from build123d import *

# Parameters (mm, degrees)
MODEL_R             = 2.5
BOSS_EXTRUDE1_DEPTH = 3


with BuildPart() as part:
    # Model → Boss-Extrude1 (new body)
    with BuildSketch(Plane.XY):
        with BuildLine():
            Line((-36.75, 0), (36.75, 0))
            ThreePointArc((36.75, 0), (40.285533906, 1.464466094), (41.75, 5))
            Line((41.75, 5), (41.75, 15))
            ThreePointArc((41.75, 15), (40.285533906, 18.535533906), (36.75, 20))
            Line((36.75, 20), (16.321067812, 20))
            ThreePointArc((16.321067812, 20), (14.40765065, 20.380602337), (12.785533906, 21.464466094))
            Line((12.785533906, 21.464466094), (3.214466094, 31.035533906))
            ThreePointArc((3.214466094, 31.035533906), (2.130602337, 32.65765065), (1.75, 34.571067812))
            Line((1.75, 34.571067812), (1.75, 45.428932188))
            ThreePointArc((1.75, 45.428932188), (2.130602337, 47.34234935), (3.214466094, 48.964466094))
            Line((3.214466094, 48.964466094), (12.785533906, 58.535533906))
            ThreePointArc((12.785533906, 58.535533906), (14.40765065, 59.619397663), (16.321067812, 60))
            Line((16.321067812, 60), (36.75, 60))
            ThreePointArc((36.75, 60), (40.285533906, 61.464466094), (41.75, 65))
            Line((41.75, 65), (41.75, 75))
            ThreePointArc((41.75, 75), (40.285533906, 78.535533906), (36.75, 80))
            Line((36.75, 80), (2.371320344, 80))
            ThreePointArc((2.371320344, 80), (1.797295195, 80.114180701), (1.310660172, 80.439339828))
            Line((1.310660172, 80.439339828), (-17.810660172, 99.560660172))
            ThreePointArc((-17.810660172, 99.560660172), (-18.135819299, 100.047295195), (-18.25, 100.621320344))
            Line((-18.25, 100.621320344), (-18.25, 123.5))
            ThreePointArc((-18.25, 123.5), (-18.689339828, 124.560660172), (-19.75, 125))
            Line((-19.75, 125), (-36.75, 125))
            ThreePointArc((-36.75, 125), (-37.810660172, 124.560660172), (-38.25, 123.5))
            Line((-38.25, 123.5), (-38.25, 1.5))
            ThreePointArc((-38.25, 1.5), (-37.810660172, 0.439339828), (-36.75, 0))
        make_face()
        with Locations((-28.25, 70)):
            Circle(MODEL_R, mode=Mode.SUBTRACT)
        with Locations((-8.25, 30)):
            Circle(MODEL_R, mode=Mode.SUBTRACT)
        with Locations((-8.25, 50)):
            Circle(MODEL_R, mode=Mode.SUBTRACT)
        with Locations((11.75, 70)):
            Circle(MODEL_R, mode=Mode.SUBTRACT)
        with Locations((31.75, 70)):
            Circle(MODEL_R, mode=Mode.SUBTRACT)
        with Locations((31.75, 10)):
            Circle(MODEL_R, mode=Mode.SUBTRACT)
        with Locations((11.75, 10)):
            Circle(MODEL_R, mode=Mode.SUBTRACT)
        with Locations((-28.25, 10)):
            Circle(MODEL_R, mode=Mode.SUBTRACT)
        with Locations((-28.25, 110)):
            Circle(MODEL_R, mode=Mode.SUBTRACT)
        with BuildLine():
            Line((-34.25, 119.15), (-34.25, 117.03))
            ThreePointArc((-34.25, 117.03), (-33.828233765, 116.011766235), (-32.81, 115.59))
            Line((-32.81, 115.59), (-23.69, 115.59))
            ThreePointArc((-23.69, 115.59), (-22.671766235, 116.011766235), (-22.25, 117.03))
            Line((-22.25, 117.03), (-22.25, 119.15))
            ThreePointArc((-22.25, 119.15), (-22.671766235, 120.168233765), (-23.69, 120.59))
            Line((-23.69, 120.59), (-32.81, 120.59))
            ThreePointArc((-32.81, 120.59), (-33.828233765, 120.168233765), (-34.25, 119.15))
        make_face(mode=Mode.SUBTRACT)
    extrude(amount=BOSS_EXTRUDE1_DEPTH)


solid = part.part
Geometry: final body of the model. Coordinates: model frame, mm. A direction names the side the tool comes from. Round coordinates to 2 decimals unless told otherwise and drop trailing zeros. Order: outer loops, then holes, each group sorted by start corner. A loop starts at its lowest first (then second) coordinate and runs counter-clockwise, first axis right, second up. Notation, with made-up numbers: (-34, -28.75) - (-13, -28.75) arc R11 ccw to (-13, -16.75) - close; hole circle Ø11 at (-36, 43.5). An arc over 180 degrees is marked (long way). Write each question's results on one line, items separated by ' | '.
Item 1: First-contact query: pin 1 Ø4 at (x, y) = (-28.25, 10) entering from -Z; pin 2 Ø1.5 at (x, z) = (17, 2) entering from +Y. Flat tips, straight axial feed; report the tip coordinate or a pass-through.
Completed:
pin 1: through | pin 2: y = 80
Item 2: Mould query, pull axis Y, two halves, no side actions, for faces 1 (the flat face through (-38.25, 63, 1)), 2 (the flat face through (-28, 125, 1)), 3 (the cylindrical face through (-8.79, 47.56, 1.48)). Classes: pulls with the +Y half, pulls with the -Y half, needs draft (parallel to the pull), parting line crosses it, or undercut.
Completed:
face 1: needs draft | face 2: pulls with the +Y half | face 3: undercut
Item 3: Material intervals for line 1 along Y through (x, z) = (31.75, 1.6); line 2 along X through (y, z) = (118.5, 0.3); line 3 along Y through (x, z) = (-24.5, 1.45), sorted ascending. Write a range as [from, to].
Completed:
line 1: [0, 7.5], [12.5, 20], [60, 67.5], [72.5, 80] | line 2: [-38.25, -34.25], [-22.25, -18.25] | line 3: [0, 115.59], [120.59, 125]
Item 4: Section A-A, the plane x = 26.5. Return the cut outline in (y, z), and give its area (3 significant figures).
Completed:
outline: (0, 0) - (20, 0) - (20, 3) - (0, 3) - close; (60, 0) - (80, 0) - (80, 3) - (60, 3) - close | area: 120 mm^2
Item 5: Section C-C, the plane y = 10. Return the cut outline in (x, z), and give its area (3 significant figures).
Completed:
outline: (-38.25, 0) - (-30.75, 0) - (-30.75, 3) - (-38.25, 3) - close; (-25.75, 0) - (9.25, 0) - (9.25, 3) - (-25.75, 3) - close; (14.25, 0) - (29.25, 0) - (29.25, 3) - (14.25, 3) - close; (34.25, 0) - (41.75, 0) - (41.75, 3) - (34.25, 3) - close | area: 195 mm^2
Item 6: Reachability of faces 4 (the flat face through (27, 20, 1)), 5 (the flat face through (-28, 120.59, 1)), 6 (the flat face through (20, 80, 1)), 7 (the cylindrical face through (40.25, 1.43, 1.48)) from +Z, -Z, +X, -X, +Y, -Y: full face, straight path, thin tool, end or side. Return the list, or none.
Completed:
face 4: +Z, -Z, +X | face 5: +Z, -Z | face 6: +Z, -Z, +X, +Y | face 7: +Z, -Z, +X, -Y
Item 7: Section B-B, the plane y = 110. Return the cut outline in (x, z), and give its area (3 significant figures).
Completed:
outline: (-38.25, 0) - (-30.75, 0) - (-30.75, 3) - (-38.25, 3) - close; (-25.75, 0) - (-18.25, 0) - (-18.25, 3) - (-25.75, 3) - close | area: 45.0 mm^2
Item 8: Section D-D, the plane x = -28.25. Return the cut outline in (y, z).
Completed:
outline: (0, 0) - (7.5, 0) - (7.5, 3) - (0, 3) - close; (12.5, 0) - (67.5, 0) - (67.5, 3) - (12.5, 3) - close; (72.5, 0) - (107.5, 0) - (107.5, 3) - (72.5, 3) - close; (112.5, 0) - (115.59, 0) - (115.59, 3) - (112.5, 3) - close; (120.59, 0) - (125, 0) - (125, 3) - (120.59, 3) - close
